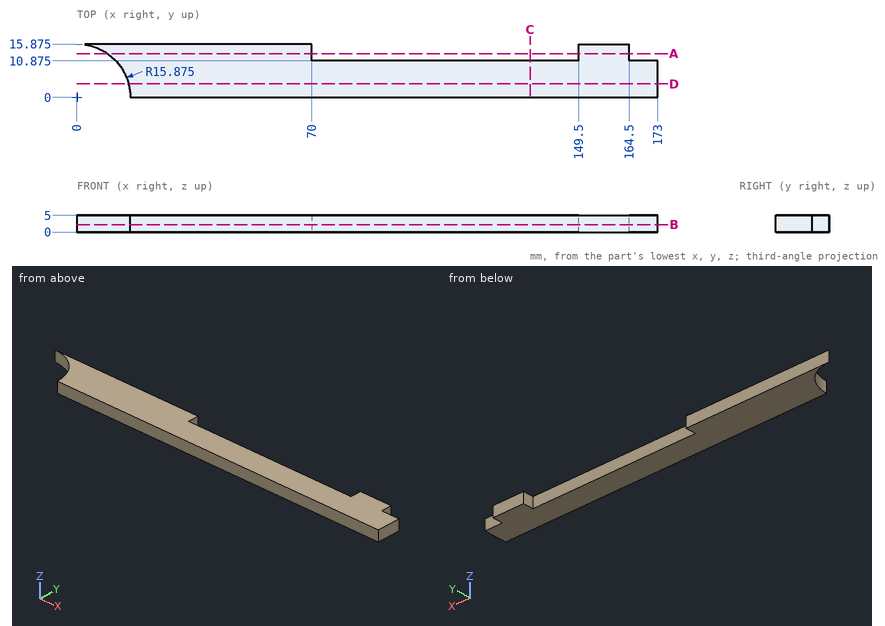
The figure shows three views and two pictorial views of one solid part (mm, origin at its lowest corner). Answer the questions. Coordinates: 2 decimals unless noted, no trailing zeros. Write each loop counter-clockwise with the first axis right and the second up, starting at its lowest first coordinate (ties: lowest second). Pieces come first, ordered by that corner, then holes. Notation, with made-up numbers: (-8, 13.5) -> (23, 13.5) arc R13 ccw to (23, 29.5) -> close; hole circle Ø2 at (-37, 5). An arc over 180 degrees is marked (long way). Return JSON: item names as keys, results as strings.
(1) The part is cut by section C-C on x = 135. Give the vertices of the cut face in (y, z) (3 decimals).
Answers below:
{"outline": "(0, 0) -> (10.875, 0) -> (10.875, 5) -> (0, 5) -> close"}
(2) The part is cut by section D-D on y = 4. Give the vertices of the cut face in (x, z), then the cut area to 3 significant figures.
Answers below:
{"outline": "(15.36, 0) -> (173, 0) -> (173, 5) -> (15.36, 5) -> close", "area": "788 mm^2"}
(3) Each of these flat-tipped pins is pushed along its axis until it touches: P1, Ø2, axis at x = 77.5, z = 1.5, coming from the +Y side (3 decimals); P2, Ø3, axis at y = 9.5, z = 3.5, coming from the -X side. Where does it stop, or does it pass through?
Answers below:
{"P1": "y = 10.875", "P2": "x = 11.45"}
(4) The part is cut by section B-B on z = 2.2. Give the vertices of the cut face in (x, y) (3 decimals).
Answers below:
{"outline": "(0, 15.875) arc R15.875 cw to (15.875, 0) -> (173, 0) -> (173, 10.875) -> (164.5, 10.875) -> (164.5, 15.875) -> (149.5, 15.875) -> (149.5, 10.875) -> (70, 10.875) -> (70, 15.875) -> close"}
(5) Consider line 1 along Y through (x, z) = (87.5, 1.1) (3 decimals); line 2 along X through (y, z) = (12.25, 3.1); line 3 along X through (y, z) = (1, 0.5). Determine where each line is inside the solid, lowest interval first. Write a range as from..to.
Answers below:
{"line 1": "0..10.875", "line 2": "10.1..70, 149.5..164.5", "line 3": "15.84..173"}
(6) The part is cut by section A-A on y = 13. Give the vertices of the cut face in (x, z).
Answers below:
{"outline": "(9.11, 0) -> (70, 0) -> (70, 5) -> (9.11, 5) -> close; (149.5, 0) -> (164.5, 0) -> (164.5, 5) -> (149.5, 5) -> close"}
